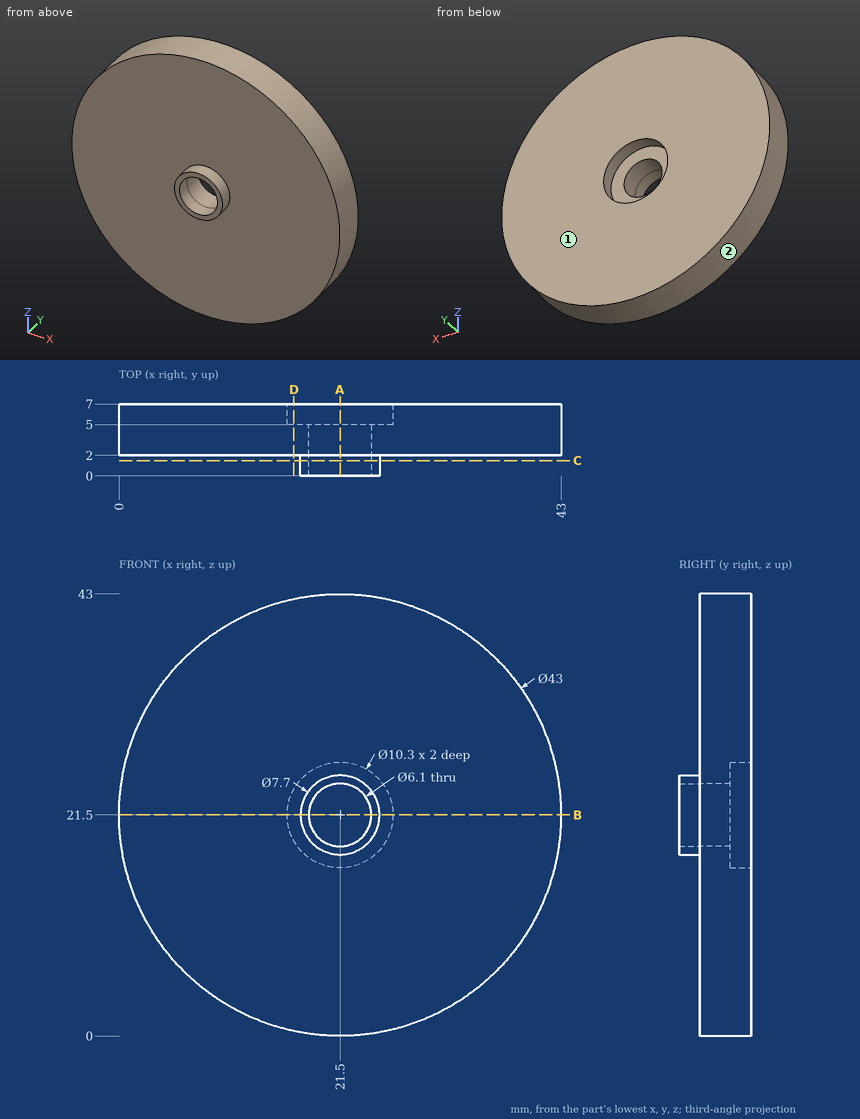
Could you check a few things on this drawing? It's one solid part, dimensions in mm from its lowest x, y, z. Round coordinates to 2 decimals unless told otherwise and drop trailing zeros. Order: outer loops, then holes, each group sorted by start corner. A loop starts at its lowest first (then second) coordinate and runs counter-clockwise, first axis right, second up.
Q1. Imagine slicing it at A-A, the plane x = 21.5. List the corners of the cut face in (y, z) for me, then the cut area to 3 significant figures.
Geometry says:
outline: (0, 17.65) - (2, 17.65) - (2, 0) - (7, 0) - (7, 16.35) - (5, 16.35) - (5, 18.45) - (0, 18.45) - close; (0, 24.55) - (5, 24.55) - (5, 26.65) - (7, 26.65) - (7, 43) - (2, 43) - (2, 25.35) - (0, 25.35) - close
area: 179 mm2
Q2. Imagine slicing it at C-C, the plane y = 1.5. List the corners of the cut face in (x, z) for me, then the cut area to 3 significant figures.
Geometry says:
outline: circle Ø7.7 at (21.5, 21.5); hole circle Ø6.1 at (21.5, 21.5)
area: 17.3 mm2
Q3. Imagine slicing it at B-B, the plane z = 21.5. List the corners of the cut face in (x, y) for me, then the cut area to 3 significant figures.
Geometry says:
outline: (0, 2) - (17.65, 2) - (17.65, 0) - (18.45, 0) - (18.45, 5) - (16.35, 5) - (16.35, 7) - (0, 7) - close; (24.55, 0) - (25.35, 0) - (25.35, 2) - (43, 2) - (43, 7) - (26.65, 7) - (26.65, 5) - (24.55, 5) - close
area: 179 mm2
Q4. Imagine slicing it at D-D, the plane x = 17. List the corners of the cut face in (y, z) for me, then the cut area to 3 significant figures.
Geometry says:
outline: (2, 0.48) - (7, 0.48) - (7, 19) - (5, 19) - (5, 24) - (7, 24) - (7, 42.52) - (2, 42.52) - close
area: 200 mm2
Q5. Thinking about a two-plate mould opening in Z: for the marked faces 1 and 2, which applies, released by +Z, released by -Z, zero draft, split by the parting line, or undercut?
Geometry says:
face 1: zero draft
face 2: split by the parting line
Q6. I'm going to push flat-ended pins straight in: P1, Ø5.5, axis at x = 21.5, z = 21.5, coming from the -Y side; P2, Ø2, axis at x = 13, z = 20.5, coming from the -Y side; P3, Ø4, axis at x = 13.5, y = 3, coming from the -Z side. Where does each tip first touch, or does it pass through?
Geometry says:
P1: passes through
P2: stops at y = 2
P3: stops at z = 0.85
Q7. Please list where these lines run through material, in increasing order: probe 1 along Z at (x, y) = (21.5, 0.9); probe 2 along Z at (x, y) = (21.5, 3.55); probe 3 along Y at (x, z) = (28, 7).
Geometry says:
probe 1: z = 17.65 to 18.45, 24.55 to 25.35
probe 2: z = 0 to 18.45, 24.55 to 43
probe 3: y = 2 to 7
